Source: three-view drawing plus pictorial views. Frame: mm from the lowest corner of the part. A direction names the side the tool comes from. Give positions to 0.01 mm unless a question says otherwise; leave off trailing zeros. Loops run counter-clockwise (first coordinate to the right, second up) from the corner with the lowest first, then second, coordinate; pieces in that order, holes last. Notation, with made-up numbers: M -4,12 L 5,12 A24 cw 5,44 Z; hole C 71.25,19.25 d6. An arc over 180 degrees is marked long. One line per item, written item: value. Start each with the question number.
(1) Section B-B on x = 44.45. Output: boundary loops of the cut face in (y, z) (1 decimal).
(2) Section C-C on y = 7.75. Output: boundary loops of the cut face in (x, z).
(3) Pin query (flat end, axial travel): P1, Ø3, axis at y = 12, z = 16, coming from the -X side; P2, Ø10, axis at x = 25, z = 15.5, coming from the +Y side; P3, Ø6, axis at x = 6.35, y = 12.7, coming from the +Z side. Return the tip coordinate at first contact, or that it passes through.
(4) Access query for the marked faces 5, 6, 7 and 8. Directions: +Z, -Z, +X, -X, +Y, -Y. A direction counts if a zero-diameter tool reaches every point of the face in a straight line with its end or side. Return the directions, or none.
(5) Ray query, line 1 along Y through (x, z) = (6.35, 2.75) (1 decimal); line 2 along Z through (x, y) = (25.4, 14); line 3 along X through (y, z) = (13, 7.25). Return the intervals inside material, ascending. Write a range as from..to.
(6) Pull-direction query (Z, two-part tool) for the marked faces 1, 2, 3 and 4; classes: released by +Z, released by -Z, zero draft, split by the parting line, or undercut.
(7) Section A-A on y = 12.7. Output: boundary loops of the cut face in (x, z) (1 decimal).
(8) Section D-D on z = 2.5. State how many separate pieces and enclosed holes the cut face has, plus the area to 3 significant figures.
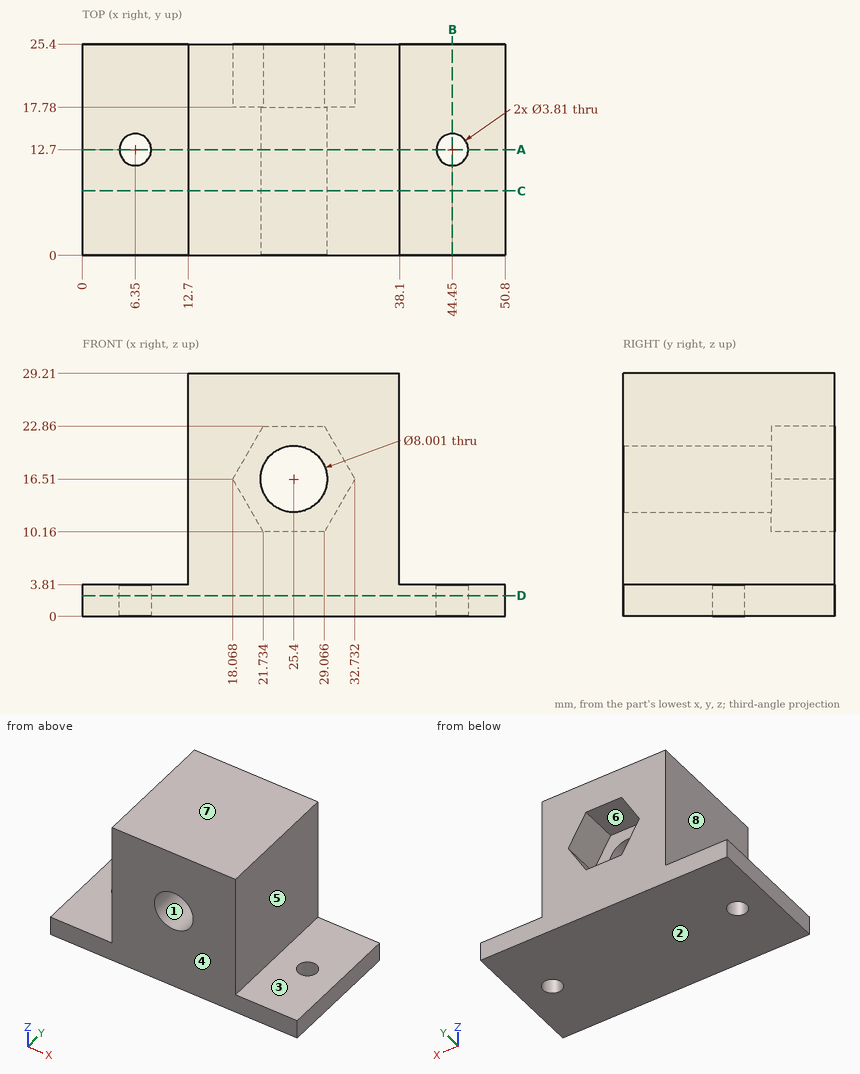
Output values:
1. outline: M 0,0 L 10.8,0 L 10.8,3.8 L 0,3.8 Z; M 14.6,0 L 25.4,0 L 25.4,3.8 L 14.6,3.8 Z
2. outline: M 0,0 L 50.8,0 L 50.8,3.81 L 38.1,3.81 L 38.1,29.21 L 12.7,29.21 L 12.7,3.81 L 0,3.81 Z; hole C 25.4,16.51 d8
3. P1: stops at x = 12.7
3. P2: stops at y = 17.78
3. P3: stops at z = 3.81
4. face 5: +Z, +X, +Y, -Y
4. face 6: +Y
4. face 7: +Z, +X, -X, +Y, -Y
4. face 8: +Z, -X, +Y, -Y
5. line 1: y = 0..10.8, 14.6..25.4
5. line 2: z = 0..12.51, 20.51..29.21
5. line 3: x = 12.7..38.1
6. face 1: undercut
6. face 2: released by -Z
6. face 3: released by +Z
6. face 4: zero draft
7. outline: M 0,0 L 4.4,0 L 4.4,3.8 L 0,3.8 Z; M 8.3,0 L 42.5,0 L 42.5,3.8 L 38.1,3.8 L 38.1,29.2 L 12.7,29.2 L 12.7,3.8 L 8.3,3.8 Z; M 46.4,0 L 50.8,0 L 50.8,3.8 L 46.4,3.8 Z; hole C 25.4,16.5 d8
8. separate pieces: 1
8. enclosed holes: 2
8. area: 1,270 mm²
